Part print with two shaded views. Sizes in mm from the minimum x, y, z corner. A direction names the side the tool comes from. Round coordinates to 2 decimals unless told otherwise and drop trailing zeros. Write each loop counter-clockwise with the first axis right and the second up, starting at its lowest first coordinate (ties: lowest second). Pieces come first, ordered by that corner, then holes. Notation, with made-up numbers: (-3.75, -33.5) - (22.25, -33.5) arc R31 cw to (22.25, -9.5) - close; hole circle Ø7 at (-6.75, -25.5). An arc over 180 degrees is marked (long way). Use one line per item in the form item = value. Start each with the question number.
Item 1: Band-saw the part on A-A, the plane y = 12. List the corners of the cut face in (x, z), and give its area (3 significant figures).
Item 2: Tool access for the marked faces 5 and 6: list every direction of +Z, -Z, +X, -X, +Y, -Y with a clear straight run to the whole face (end or side of a thin tool).
Item 3: Band-saw the part on C-C, the plane x = 11. List the corners of the cut face in (y, z) (3 decimals), and give its area (3 significant figures).
Item 4: Pull direction Z, two halves, no side cores. Call the marked faces 1, 2, 3 and 4: +Z half, -Z half, draft (parallel to the pull), parting line (faces both ways), or undercut.
Item 5: Band-saw the part on B-B, the plane y = 15.24. List the corners of the cut face in (x, z).
Item 6: Pin check, flat tips, straight feed: pin 1 (0.7 mm diameter, centred on y = 0.5, z = 4.5, fed in from -X); pin 2 (0.5 mm diameter, centred on x = 0.5, z = 2, fed in from -Y). Stop position of each tip, or through.
Item 7: Drill centre lines: L1, parallel to X at y = 9.5, z = 3; L2, parallel to Y at x = 7.25, z = 1 (3 decimals); L3, parallel to Y at x = 3.75, z = 4.5 (3 decimals). Where is each one in solid material? Low to high.
Item 8: Band-saw the part on D-D, the plane z = 3.75. List the corners of the cut face in (x, y) (3 decimals).
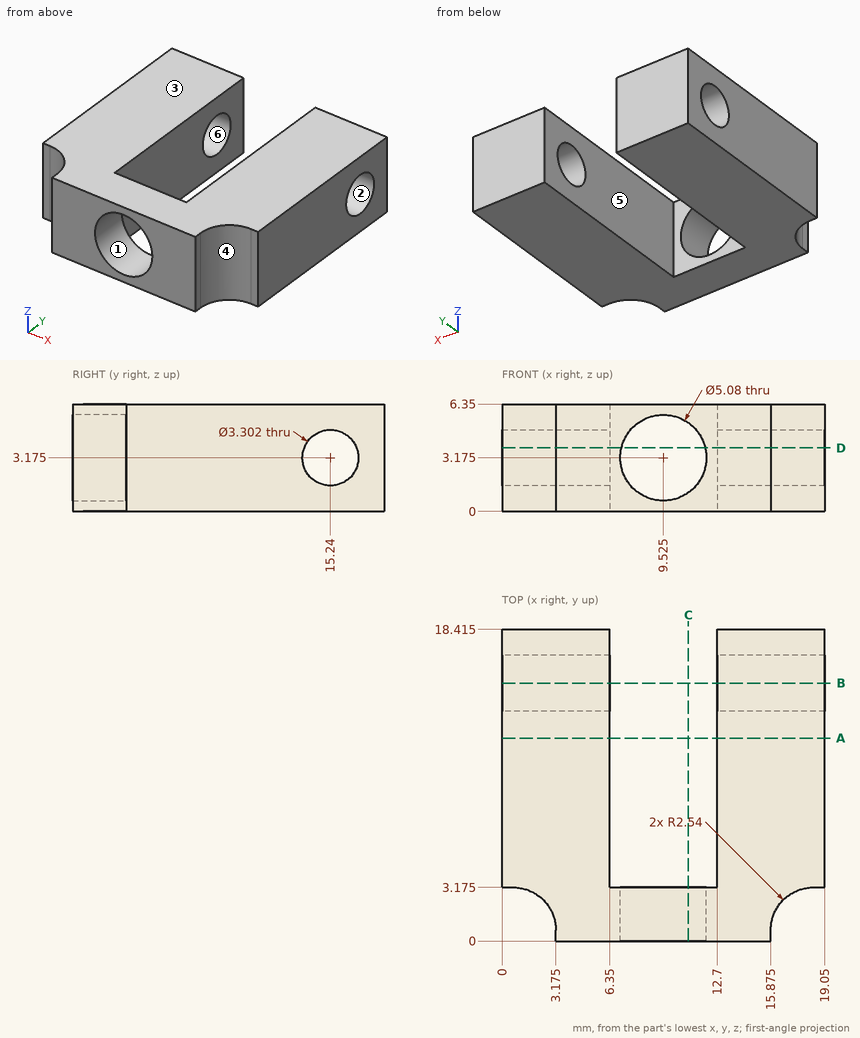
Determined:
q1.outline = (0, 0) - (6.35, 0) - (6.35, 6.35) - (0, 6.35) - close; (12.7, 0) - (19.05, 0) - (19.05, 6.35) - (12.7, 6.35) - close
q1.area = 80.6 mm²
q2.face_5 = +Z, -Z, +Y
q2.face_6 = +X, -X
q3.outline = (0, 0) - (3.175, 0) - (3.175, 1.107) - (0, 1.107) - close; (0, 5.243) - (3.175, 5.243) - (3.175, 6.35) - (0, 6.35) - close
q3.area = 7.03 mm²
q4.face_1 = undercut
q4.face_2 = undercut
q4.face_3 = +Z half
q4.face_4 = draft
q5.outline = (0, 0) - (6.35, 0) - (6.35, 1.52) - (0, 1.52) - close; (0, 4.83) - (6.35, 4.83) - (6.35, 6.35) - (0, 6.35) - close; (12.7, 0) - (19.05, 0) - (19.05, 1.52) - (12.7, 1.52) - close; (12.7, 4.83) - (19.05, 4.83) - (19.05, 6.35) - (12.7, 6.35) - close
q6.pin_1 = 3.17
q6.pin_2 = 3.17
q7.L1 = 0 to 6.35, 12.7 to 19.05
q7.L2 = 0 to 3.175
q7.L3 = 0 to 14.255, 16.225 to 18.415
q8.outline = (0, 3.175) - (0.635, 3.175) arc R2.54 cw to (3.175, 0.635) - (3.175, 0) - (7.051, 0) - (7.051, 3.175) - (6.35, 3.175) - (6.35, 13.692) - (0, 13.692) - close; (0, 16.788) - (6.35, 16.788) - (6.35, 18.415) - (0, 18.415) - close; (11.999, 0) - (15.875, 0) - (15.875, 0.635) arc R2.54 cw to (18.415, 3.175) - (19.05, 3.175) - (19.05, 13.692) - (12.7, 13.692) - (12.7, 3.175) - (11.999, 3.175) - close; (12.7, 16.788) - (19.05, 16.788) - (19.05, 18.415) - (12.7, 18.415) - close
